Here's how the part is built. I have some questions about the finished solid (model axes, mm). Face numbers are marked on the shaded views. A direction names the side the tool comes from. Coordinates: 2 decimals unless noted, no trailing zeros. Write each loop counter-clockwise with the first axis right and the second up, starting at its lowest first coordinate (ties: lowest second). Pieces come first, ordered by that corner, then holes. Notation, with made-up numbers: (-9, 72) -> (21, 72) arc R29 cw to (21, 96) -> close; hole circle Ø8 at (77.25, 83). An arc over 180 degrees is marked (long way). Use CSV: the item, a comma, the result in double quotes. Start each with the question number.
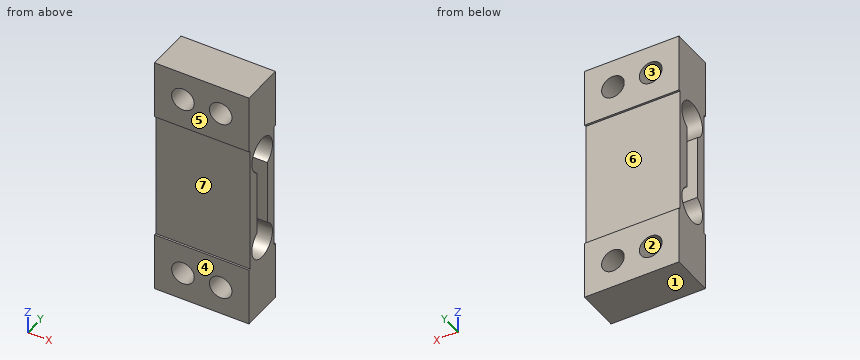
```python
from build123d import *

# Parameters (mm, degrees)
SKETCH2_W           = 130
SKETCH2_H           = 23
BOSS_EXTRUDE1_DEPTH = 50
SKETCH3_R           = 6
CUT_EXTRUDE1_DEPTH  = 23
SKETCH4_W           = 50
SKETCH4_H           = 68
CUT_EXTRUDE3_DEPTH  = 1
SKETCH5_W           = 50
SKETCH5_H           = 68
CUT_EXTRUDE4_DEPTH  = 1


with BuildPart() as part:
    # Sketch2 → Boss-Extrude1 (new body)
    with BuildSketch(Plane(origin=(0, 0, 0), x_dir=(0, 0, -1), z_dir=(1, 0, 0))):
        with Locations((65, 11.5)):
            Rectangle(SKETCH2_W, SKETCH2_H)
        with BuildLine():
            Line((82.205771366, 16), (47.794228634, 16))
            ThreePointArc((47.794228634, 16), (31, 11.5), (47.794228634, 7))
            Line((47.794228634, 7), (82.205771366, 7))
            ThreePointArc((82.205771366, 7), (99, 11.5), (82.205771366, 16))
        make_face(mode=Mode.SUBTRACT)
    extrude(amount=BOSS_EXTRUDE1_DEPTH)

    # Sketch3 → Cut-Extrude1 (cut)
    with BuildSketch(Plane(origin=(0, 23, 0), x_dir=(1, 0, 0), z_dir=(0, 1, 0))):
        with Locations((15, 15)):
            Circle(SKETCH3_R)
        with Locations((35, 15)):
            Circle(SKETCH3_R)
        with Locations((15, 115)):
            Circle(SKETCH3_R)
        with Locations((35, 115)):
            Circle(SKETCH3_R)
    extrude(amount=-CUT_EXTRUDE1_DEPTH, mode=Mode.SUBTRACT)

    # Sketch4 → Cut-Extrude3 (cut)
    with BuildSketch(Plane(origin=(0, 23, 0), x_dir=(1, 0, 0), z_dir=(0, 1, 0))):
        with Locations((25, 65)):
            Rectangle(SKETCH4_W, SKETCH4_H)
    extrude(amount=-CUT_EXTRUDE3_DEPTH, mode=Mode.SUBTRACT)

    # Sketch5 → Cut-Extrude4 (cut)
    with BuildSketch(Plane.XZ):
        with Locations((25, -65)):
            Rectangle(SKETCH5_W, SKETCH5_H)
    extrude(amount=-CUT_EXTRUDE4_DEPTH, mode=Mode.SUBTRACT)


solid = part.part
```
Item 1: Which directions (+Z, -Z, +X, -X, +Y, -Y) give clear straight access to the entire face, cutting with the end or side of a thin tool? Please do the marked faces 5, 6 and 7.
Item 2: If I drill on line 1 along X through (y, z) = (5.75, -115); line 2 along Y through (x, z) = (5.5, -67); line 3 along Z through (x, y) = (15, 7.5), over which ranges is the centre line in solid material (lowest first)?
Item 3: I want a section at D-D on z = -115. Please give me the cut outline in (x, y).
Item 4: I want a section at B-B on y = 11.5. Please give me the cut outline in (x, z), then the cut area to 3 significant figures.
Item 5: I want a section at A-A on z = -90. Please give me the cut outline in (x, y), then the cut area to 3 significant figures.
Item 6: I want a section at C-C on x = 35. Please give me the cut outline in (y, z).
Item 7: I'm going to push flat-ended pins straight in: pin 1 (2 mm diameter, centred on x = 11.5, z = -16, fed in from +Y); pin 2 (5 mm diameter, centred on y = 16, z = -82.5, fed in from -X); pin 3 (4 mm diameter, centred on x = 33.5, z = -68.5, fed in from -Y); pin 4 (12 mm diameter, centred on x = 18.5, z = -71.5, fed in from +Y). Where does each tip first touch, or does it pass through?
Item 8: Thinking about a two-plate mould opening in Z: for the marked faces 1, 2, 3 and 4, which applies, +Z half, -Z half, draft (parallel to the pull), parting line (faces both ways), or undercut?
Geometry says:
1,face 5,"+Z, -Z, +X, -X, -Y"
1,face 6,"+X, -X, +Y"
1,face 7,"+X, -X, -Y"
2,line 1,"0 to 9, 21 to 29, 41 to 50"
2,line 2,"1 to 7, 16 to 22"
2,line 3,"-130 to -121, -109 to -98.06, -31.94 to -21, -9 to 0"
3,outline,"(0, 0) -> (9, 0) -> (9, 23) -> (0, 23) -> close; (21, 0) -> (29, 0) -> (29, 23) -> (21, 23) -> close; (41, 0) -> (50, 0) -> (50, 23) -> (41, 23) -> close"
4,outline,"(0, -130) -> (50, -130) -> (50, -99) -> (0, -99) -> close; (0, -31) -> (50, -31) -> (50, 0) -> (0, 0) -> close; hole circle Ø12 at (15, -115); hole circle Ø12 at (15, -15); hole circle Ø12 at (35, -115); hole circle Ø12 at (35, -15)"
4,area,"2,650 mm2"
5,outline,"(0, 1) -> (50, 1) -> (50, 2.5) -> (0, 2.5) -> close; (0, 20.5) -> (50, 20.5) -> (50, 22) -> (0, 22) -> close"
5,area,"150 mm2"
6,outline,"(0, -130) -> (23, -130) -> (23, -121) -> (0, -121) -> close; (0, -109) -> (23, -109) -> (23, -99) -> (22, -99) -> (22, -31) -> (23, -31) -> (23, -21) -> (0, -21) -> (0, -31) -> (1, -31) -> (1, -99) -> (0, -99) -> close; (0, -9) -> (23, -9) -> (23, 0) -> (0, 0) -> close; hole (7, -82.21) arc R9 ccw (long way) to (16, -82.21) -> (16, -47.79) arc R9 ccw (long way) to (7, -47.79) -> close"
7,pin 1,"through"
7,pin 2,"x = 0"
7,pin 3,"y = 1"
7,pin 4,"y = 22"
8,face 1,"-Z half"
8,face 2,"undercut"
8,face 3,"undercut"
8,face 4,"draft"
